Geometry check sheet. Reference: the model listing, model coordinates, mm. Face numbers are marked on the shaded views. Round coordinates to 2 decimals unless told otherwise and drop trailing zeros. Order: outer loops, then holes, each group sorted by start corner. A loop starts at its lowest first (then second) coordinate and runs counter-clockwise, first axis right, second up. Notation, with made-up numbers: (76, -24.75) -> (120, -24.75) arc R11 ccw to (120, -3.75) -> close; hole circle Ø11 at (13.5, 2.25). An arc over 180 degrees is marked (long way). Use a Markdown table: item, result. Add a question column.
Item 1: Sectioned sample at C-C, the plane x = 20.75. Record the cut outline in (y, z).
Item 2: Mould release check, pull along X, two halves, no side actions. Record for the marked faces 1, 2, 3 and 4: pulls with the +X half, pulls with the -X half, needs draft (parallel to the pull), parting line crosses it, or undercut.
Item 3: Sectioned sample at B-B, the plane y = -7. Record the cut outline in (x, z).
Item 4: Gauge pin test, flat ends, axial feed: pin 1 Ø1.5 at (x, y) = (23, -10) entering from +Z; pin 2 Ø1.5 at (x, z) = (5.5, 10.5) entering from -Y; pin 3 Ø3 at (y, z) = (-21, 15.5) entering from -X. Record the tip position at first contact, or that the pin passes through.
Item 5: Sectioned sample at A-A, the plane z = 11. Record the cut outline in (x, y).
Item 6: Sectioned sample at D-D, the plane y = -20. Record the cut outline in (x, z).
Item 7: Material ranges on probe 1 along Y at (x, z) = (11.25, 9); probe 2 along X at (y, z) = (-10, 5.75); probe 3 along Z at (x, y) = (10.5, -17), recorded low to high. Write a range as [from, to].
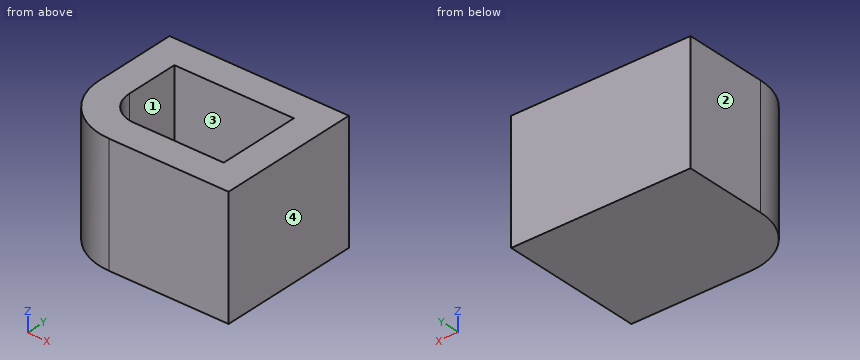
from build123d import *

# Parameters (mm, degrees)
F0_W     = 30
F0_H     = 20
F1_DEPTH = 24
F2_R     = 10
F3_T     = -5


with BuildPart() as f1:
    # F0 (on Front) → F1 (new body)
    with BuildSketch(Plane.XZ):
        with Locations((15, 10)):
            Rectangle(F0_W, F0_H)
    extrude(amount=F1_DEPTH)

    # F2
    f2_edges = [f1.edges().sort_by_distance(p)[0] for p in [
        (0, -24, 10),
    ]]
    fillet(f2_edges, radius=F2_R)

    # F3
    f3_openings = [f1.faces().sort_by_distance(p)[0] for p in [
        (15.3922, -11.699964, 20),
    ]]
    offset(amount=F3_T, openings=f3_openings)


solid = f1.part
Found:
| question | item | result |
|---|---|---|
| 1 | outline | (-24, 0) -> (0, 0) -> (0, 20) -> (-5, 20) -> (-5, 5) -> (-19, 5) -> (-19, 20) -> (-24, 20) -> close |
| 2 | face 1 | undercut |
| 2 | face 2 | pulls with the -X half |
| 2 | face 3 | undercut |
| 2 | face 4 | pulls with the +X half |
| 3 | outline | (0, 0) -> (30, 0) -> (30, 20) -> (25, 20) -> (25, 5) -> (5, 5) -> (5, 20) -> (0, 20) -> close |
| 4 | pin 1 | stops at z = 5 |
| 4 | pin 2 | stops at y = -23.27 |
| 4 | pin 3 | stops at x = 1.65 |
| 5 | outline | (0, -14) arc R10 ccw to (10, -24) -> (30, -24) -> (30, 0) -> (0, 0) -> close; hole (5, -14) arc R5 ccw to (10, -19) -> (25, -19) -> (25, -5) -> (5, -5) -> close |
| 6 | outline | (2, 0) -> (30, 0) -> (30, 20) -> (2, 20) -> close |
| 7 | probe 1 | y = [-24, -19], [-5, 0] |
| 7 | probe 2 | x = [0, 5], [25, 30] |
| 7 | probe 3 | z = [0, 5] |
